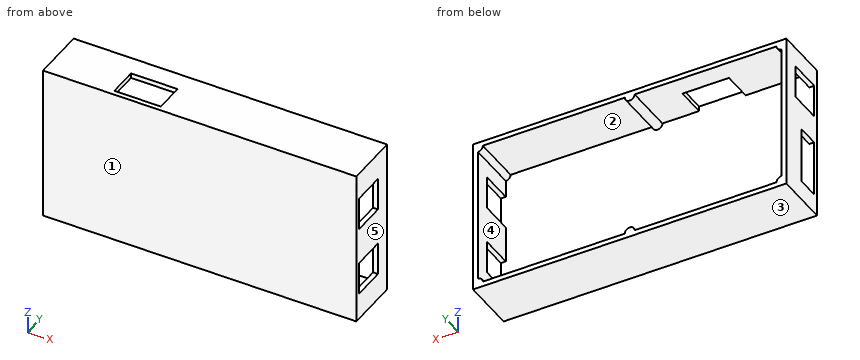
from build123d import *

# Parameters (mm, degrees)
SKETCH3_W           = 128
SKETCH3_H           = 64
BOSS_EXTRUDE1_DEPTH = 22
BOSS_EXTRUDE3_DEPTH = 2
CUT_EXTRUDE1_REACH  = 130
SKETCH5_W           = 13.5
SKETCH5_H           = 13.5
SKETCH6_W           = 23
SKETCH6_H           = 9
SKETCH6_W_2         = 13.5
SKETCH6_H_2         = 13.5
CUT_EXTRUDE2_DEPTH  = 2
SKETCH7_W           = 19
SKETCH7_H           = 12
CUT_EXTRUDE3_DEPTH  = 2


with BuildPart() as part:
    # Sketch3 → Boss-Extrude1 (new body)
    with BuildSketch(Plane(origin=(0, 0, 0), x_dir=(1, 0, 0), z_dir=(0, 1, 0))):
        Rectangle(SKETCH3_W, SKETCH3_H)
        with BuildLine():
            Line((60, -30), (2, -30))
            ThreePointArc((2, -30), (0, -28), (-2, -30))
            Line((-2, -30), (-60, -30))
            ThreePointArc((-60, -30), (-60.585786438, -28.585786438), (-62, -28))
            Line((-62, -28), (-62, 28))
            ThreePointArc((-62, 28), (-60.585786438, 28.585786438), (-60, 30))
            Line((-60, 30), (-2, 30))
            ThreePointArc((-2, 30), (0, 28), (2, 30))
            Line((2, 30), (60, 30))
            ThreePointArc((60, 30), (60.585786438, 28.585786438), (62, 28))
            Line((62, 28), (62, -28))
            ThreePointArc((62, -28), (60.585786438, -28.585786438), (60, -30))
        make_face(mode=Mode.SUBTRACT)
    extrude(amount=BOSS_EXTRUDE1_DEPTH)

    # Sketch3_5 → Boss-Extrude3 (add)
    with BuildSketch(Plane(origin=(0, 0, 0), x_dir=(1, 0, 0), z_dir=(0, 1, 0))):
        with BuildLine():
            ThreePointArc((62, 28), (60.585786438, 28.585786438), (60, 30))
            Line((60, 30), (2, 30))
            ThreePointArc((2, 30), (0, 28), (-2, 30))
            Line((-2, 30), (-60, 30))
            ThreePointArc((-60, 30), (-60.585786438, 28.585786438), (-62, 28))
            Line((-62, 28), (-62, -28))
            ThreePointArc((-62, -28), (-60.585786438, -28.585786438), (-60, -30))
            Line((-60, -30), (-2, -30))
            ThreePointArc((-2, -30), (0, -28), (2, -30))
            Line((2, -30), (60, -30))
            ThreePointArc((60, -30), (60.585786438, -28.585786438), (62, -28))
            Line((62, -28), (62, 28))
        make_face()
    extrude(amount=BOSS_EXTRUDE3_DEPTH)

    # Sketch5 → Cut-Extrude1 (cut, up to next)
    with BuildSketch(Plane(origin=(64, 0, 0), x_dir=(0, 0, -1), z_dir=(1, 0, 0)), mode=Mode.PRIVATE) as cut_extrude1_sk1:
        with Locations((14.25, 8.75)):
            Rectangle(SKETCH5_W, SKETCH5_H)
    cut_extrude1_tool1 = extrude(cut_extrude1_sk1.sketch, amount=-CUT_EXTRUDE1_REACH, mode=Mode.PRIVATE) & part.part
    add(cut_extrude1_tool1.solids().sort_by_distance((64, 8.75, -14.25))[0], mode=Mode.SUBTRACT)
    # Sketch5 → Cut-Extrude1 (cut, up to next)
    with BuildSketch(Plane(origin=(64, 0, 0), x_dir=(0, 0, -1), z_dir=(1, 0, 0)), mode=Mode.PRIVATE) as cut_extrude1_sk2:
        with Locations((-14.25, 8.75)):
            Rectangle(SKETCH5_W, SKETCH5_H)
    cut_extrude1_tool2 = extrude(cut_extrude1_sk2.sketch, amount=-CUT_EXTRUDE1_REACH, mode=Mode.PRIVATE) & part.part
    add(cut_extrude1_tool2.solids().sort_by_distance((64, 8.75, 14.25))[0], mode=Mode.SUBTRACT)

    # Sketch6 → Cut-Extrude2 (cut)
    with BuildSketch(Plane.ZY.offset(64)):
        with Locations((-12.5, 6.5)):
            Rectangle(SKETCH6_W, SKETCH6_H)
        with Locations((17.25, 8.75)):
            Rectangle(SKETCH6_W_2, SKETCH6_H_2)
    extrude(amount=-CUT_EXTRUDE2_DEPTH, mode=Mode.SUBTRACT)

    # Sketch7 → Cut-Extrude3 (cut)
    with BuildSketch(Plane.XY.offset(32)):
        with Locations((-26.5, 8)):
            Rectangle(SKETCH7_W, SKETCH7_H)
    extrude(amount=-CUT_EXTRUDE3_DEPTH, mode=Mode.SUBTRACT)


solid = part.part
For this review, take the finished solid that the model builds, in its own axes (mm). Face numbers are marked on the shaded views. A direction names the side the tool comes from. Round coordinates to 2 decimals unless told otherwise and drop trailing zeros. Loops run counter-clockwise (first coordinate to the right, second up) from the corner with the lowest first, then second, coordinate; pieces in that order, holes last. Notation, with made-up numbers: (50.5, -2) - (88.5, -2) arc R20 cw to (88.5, 8) - close; hole circle Ø5 at (19, -33). An arc over 180 degrees is marked (long way). One line per question, with ' | ' between items.
Q1. For line 1 along X through (y, z) = (20.5, -19); line 2 along Z through (x, y) = (-25, 20.25); line 3 along Y through (x, z) = (46, -8.5), list the stretches that pass through material, from the lowest coordinate up. Write a range as [from, to].
Taken from the geometry:
line 1: x = [-64, -62], [62, 64] | line 2: z = [-32, -30], [30, 32] | line 3: y = [0, 2]
Q2. Take a section at D-D (y = 4.5). State how many separate pieces and enclosed holes the cut face has, and give its area (3 significant figures).
Taken from the geometry:
separate pieces: 5 | enclosed holes: 0 | area: 612 mm²
Q3. Tool access review of the marked faces 4 and 5: name each direction out of +Z, -Z, +X, -X, +Y, -Y from which nothing blocks a thin tool from reaching the whole face with its end or side.
Taken from the geometry:
face 4: +Y | face 5: +Z, -Z, +X, +Y, -Y
Q4. Take a section at B-B (y = 19). Give the boundary of the cut face in (x, z).
Taken from the geometry:
outline: (-64, -32) - (64, -32) - (64, 32) - (-64, 32) - close; hole (-62, -28) arc R2 cw to (-60, -30) - (-2, -30) arc R2 cw to (2, -30) - (60, -30) arc R2 cw to (62, -28) - (62, 28) arc R2 cw to (60, 30) - (2, 30) arc R2 cw to (-2, 30) - (-60, 30) arc R2 cw to (-62, 28) - close
Q5. For pin 1 (4 mm diameter, centred on x = -15.5, z = 9, fed in from +Y), flat-tipped, find the tip position at first contact; note if it passes through.
Taken from the geometry:
pin 1: stops at y = 2
Q6. Take a section at A-A (x = 0). Give the boundary of the cut face in (y, z), and give its area (3 significant figures).
Taken from the geometry:
outline: (0, -32) - (22, -32) - (22, -28) - (2, -28) - (2, 28) - (22, 28) - (22, 32) - (0, 32) - close | area: 288 mm²
Q7. The part is to be moulded in two halves that separate along Z. For the marked faces 1, 2 and 3, say which applies: released by +Z, released by -Z, zero draft, split by the parting line, or undercut.
Taken from the geometry:
face 1: zero draft | face 2: undercut | face 3: released by -Z
Q8. Take a section at C-C (x = -53). Give the boundary of the cut face in (y, z).
Taken from the geometry:
outline: (0, -32) - (22, -32) - (22, -30) - (2, -30) - (2, 30) - (22, 30) - (22, 32) - (0, 32) - close
